Geometry check sheet. Reference: the model listing, model coordinates, mm. A direction names the side the tool comes from. Round coordinates to 2 decimals unless told otherwise and drop trailing zeros. Order: outer loops, then holes, each group sorted by start corner. A loop starts at its lowest first (then second) coordinate and runs counter-clockwise, first axis right, second up. Notation, with made-up numbers: (-27, 51.25) - (-6, 51.25) arc R20 ccw to (-6, 59.25) - close; hole circle Ø1 at (51.25, -22.75). An arc over 180 degrees is marked (long way). Use a Markdown table: item, result. Add a question column.
(1) Section check B-B on z = 41. Record the boundary of the cut face in (x, y), then the cut area to 3 significant figures.
(2) Access from +Z, -Z, +X, -X, +Y, -Y to the whole of each face (thin tool, end or side, straight path). Record for faces 4 (the face through (-5.2, 0.1, -0.8)), 5 (the face through (17, 0, -2)), 6 (the face through (11, -4, -2)), 7 (the face through (11, 4, -2)), 8 (the face through (6.5, 0.1, 0.9)).
(3) Thickness scan on line 1 along Z through (x, y) = (-5, 8.5); line 2 along X through (y, z) = (0, 53); line 3 along X through (y, z) = (8, 95.5). Record the ranges inside material, lowest first. Write a range as [from, to].
(4) Mould release check, pull along X, two halves, no side actions. Record for faces 1 (the face through (5, 0, -2)), 2 (the face through (11, 0, 133)), 3 (the face through (11, 0, 6)): released by +X, released by -X, zero draft, split by the parting line, or undercut.
(5) Gauge pin test, flat ends, axial feed: P1, Ø5, axis at y = -8, z = 109.5, coming from the -X side; P2, Ø3.5, axis at x = 10, z = -2.5, coming from the +Y side; P3, Ø1, axis at y = 8, z = 50, coming from the -X side. Record the tip position at first contact, or that the pin passes through.
(6) Section check C-C on y = 9.25. Record the boundary of the cut face in (x, z).
```python
from build123d import *

# Parameters (mm, degrees)
EXTRUSION1_DEPTH = 133
EXTRUSION2_DEPTH = 1
CHANFREIN1_SIZE  = 1
EXTRUSION3_DEPTH = 3
EXTRUSION4_DEPTH = 10


with BuildPart() as part:
    # Esquisse1 → Extrusion1 (new body)
    with BuildSketch(Plane.XY):
        with BuildLine():
            Line((0, 11.5), (22, 11.5))
            ThreePointArc((22, 11.5), (33.5, 0), (22, -11.5))
            Line((22, -11.5), (0, -11.5))
            ThreePointArc((0, -11.5), (-11.5, 0), (0, 11.5))
        make_face()
    extrude(amount=EXTRUSION1_DEPTH)

    # Esquisse2 → Extrusion2 (add)
    with BuildSketch(Plane(origin=(0, 0, 0), x_dir=(-1, 0, 0), z_dir=(0, 0, -1))):
        with BuildLine():
            Line((-22, 5), (0, 5))
            ThreePointArc((0, 5), (5, 0), (0, -5))
            Line((0, -5), (-22, -5))
            ThreePointArc((-22, -5), (-27, 0), (-22, 5))
        make_face()
    extrude(amount=EXTRUSION2_DEPTH)

    # Chanfrein1
    chanfrein1_edges = [part.edges().sort_by_distance(p)[0] for p in [
        (11, 5, 0),
        (-5, 0, 0),
        (27, 0, 0),
        (11, -5, 0),
    ]]
    chamfer(chanfrein1_edges, length=CHANFREIN1_SIZE - 0.0001)  # a hair under: the kernel refuses the full size

    # Esquisse3 → Extrusion3 (add)
    with BuildSketch(Plane(origin=(0, 0, -1), x_dir=(-1, 0, 0), z_dir=(0, 0, -1))):
        with BuildLine():
            Line((-13, 4), (-9, 4))
            ThreePointArc((-9, 4), (-5, 0), (-9, -4))
            Line((-9, -4), (-13, -4))
            ThreePointArc((-13, -4), (-17, 0), (-13, 4))
        make_face()
    extrude(amount=EXTRUSION3_DEPTH)

    # Esquisse4 → Extrusion4 (cut)
    with BuildSketch(Plane(origin=(0, 0, -4), x_dir=(-1, 0, 0), z_dir=(0, 0, -1))):
        with BuildLine():
            Line((-13, 2.5), (-9, 2.5))
            ThreePointArc((-9, 2.5), (-6.5, 0), (-9, -2.5))
            Line((-9, -2.5), (-13, -2.5))
            ThreePointArc((-13, -2.5), (-15.5, 0), (-13, 2.5))
        make_face()
    extrude(amount=-EXTRUSION4_DEPTH, mode=Mode.SUBTRACT)


solid = part.part
```
Check sheet entries:
| question | item | result |
|---|---|---|
| 1 | outline | (0, -11.5) - (22, -11.5) arc R11.5 ccw to (22, 11.5) - (0, 11.5) arc R11.5 ccw to start |
| 1 | area | 921 mm2 |
| 2 | face 4 | -Z, -X |
| 2 | face 5 | -Z, +X |
| 2 | face 6 | -Z, +X, -X, -Y |
| 2 | face 7 | -Z, +X, -X, +Y |
| 2 | face 8 | -Z |
| 3 | line 1 | z = [0, 133] |
| 3 | line 2 | x = [-11.5, 33.5] |
| 3 | line 3 | x = [-8.26, 30.26] |
| 4 | face 1 | released by -X |
| 4 | face 2 | zero draft |
| 4 | face 3 | undercut |
| 5 | P1 | stops at x = -10.1 |
| 5 | P2 | stops at y = 5.25 |
| 5 | P3 | stops at x = -8.72 |
| 6 | outline | (-6.83, 0) - (28.83, 0) - (28.83, 133) - (-6.83, 133) - close |
